Verification items for the finished model (mm, model axes). A direction names the side the tool comes from. Coordinates: 2 decimals unless noted, no trailing zeros. Loops run counter-clockwise (first coordinate to the right, second up) from the corner with the lowest first, then second, coordinate; pieces in that order, holes last. Notation, with made-up numbers: (73.5, 82) -> (118.5, 82) arc R12 cw to (118.5, 92) -> close; hole circle Ø11 at (38, -30). An arc over 180 degrees is marked (long way). Use CSV: the item, a comma, the result in double quotes. Start each with the question number.
```python
from build123d import *

# Parameters (mm, degrees)
AUFSATZ_LINEAR_AUSTRAGEN1_DEPTH            = 25
SCHNITT_LINEAR_AUSTRAGEN1_DEPTH            = 20
FASE1_SIZE                                 = 10
VERRUNDUNG1_R                              = 25
SKIZZE3_R                                  = 3.25
SCHNITT_LINEAR_AUSTRAGEN2_DEPTH            = 3.4
SKIZZE4_R                                  = 1.7
SCHNITT_LINEAR_AUSTRAGEN3_DEPTH            = 6.6
KREISMUSTER1_COUNT                         = 3
SKIZZE5_R                                  = 13
SCHNITT_LINEAR_AUSTRAGEN4_DEPTH            = 142.155942135
SKIZZE7_W                                  = 12
SKIZZE7_H                                  = 20
AUFSATZ_LINEAR_AUSTRAGEN2_DEPTH            = 10
SKIZZE9_R                                  = 1.7
SCHNITT_LINEAR_AUSTRAGEN7_DEPTH            = 78.781745931
SKIZZE8_R                                  = 3.25
SCHNITT_LINEAR_AUSTRAGEN6_DEPTH            = 3.4
SKIZZE10_R                                 = 13
SKIZZE10_R_2                               = 11
AUFSATZ_LINEAR_AUSTRAGEN3_DEPTH            = 2
SPIEGELN1_AT_THE_SECOND_PLANE_COPY_1_SKE_W = 12
SPIEGELN1_AT_THE_SECOND_PLANE_COPY_1_SKE_H = 20
SPIEGELN1_AT_THE_SECOND_PLANE_COPY_1_DEPTH = 10
SPIEGELN1_AT_THE_SECOND_PLANE_COPY_2_SKE_R = 1.7
SPIEGELN1_AT_THE_SECOND_PLANE_COPY_2_DEPTH = 78.781745931
SPIEGELN1_AT_THE_SECOND_PLANE_COPY_3_SKE_R = 3.25
SPIEGELN1_AT_THE_SECOND_PLANE_COPY_3_DEPTH = 3.4
SKIZZE11_R                                 = 1.9
SCHNITT_LINEAR_AUSTRAGEN8_DEPTH            = 10
KREISMUSTER2_COUNT                         = 4


with BuildPart() as part:
    # Skizze1 → Aufsatz-Linear austragen1 (new, symmetric)
    with BuildSketch(Plane(origin=(0, 0, 0), x_dir=(1, 0, 0), z_dir=(0, 1, 0))):
        Polygon((-60, 0), (60, 0), (60, -70), (48, -70), (48, -10), (-48, -10), (-48, -70), (-60, -70), align=None)
    extrude(amount=AUFSATZ_LINEAR_AUSTRAGEN1_DEPTH, both=True)

    # Skizze2 → Schnitt-Linear austragen1 (cut)
    with BuildSketch(Plane(origin=(0, 0, 0), x_dir=(-1, 0, 0), z_dir=(0, 0, -1))):
        with BuildLine():
            Line((-1.532970972, 2.1), (1.532970972, 2.1))
            ThreePointArc((1.532970972, 2.1), (0, -2.6), (-1.532970972, 2.1))
        make_face()
    extrude(amount=-SCHNITT_LINEAR_AUSTRAGEN1_DEPTH, mode=Mode.SUBTRACT)

    # Fase1
    fase1_edges = [part.edges().sort_by_distance(p)[0] for p in [
        (-60, 0, 0),
        (60, 0, 0),
        (48, 0, 10),
        (-48, 0, 10),
    ]]
    chamfer(fase1_edges, length=FASE1_SIZE)

    # Verrundung1
    verrundung1_edges = [part.edges().sort_by_distance(p)[0] for p in [
        (-54, -25, 70),
        (-54, 25, 70),
        (54, 25, 70),
        (54, -25, 70),
    ]]
    fillet(verrundung1_edges, radius=VERRUNDUNG1_R - 0.0001)  # a hair under: the kernel refuses the full size

    # Skizze3 → Schnitt-Linear austragen2 (cut)
    with BuildSketch(Plane.XY.offset(10)):
        with Locations((0, 12)):
            Circle(SKIZZE3_R)
    schnitt_linear_austragen2 = extrude(amount=-SCHNITT_LINEAR_AUSTRAGEN2_DEPTH, mode=Mode.SUBTRACT)

    # Skizze4 → Schnitt-Linear austragen3 (cut)
    with BuildSketch(Plane.XY.offset(6.6)):
        with Locations((0, 12)):
            Circle(SKIZZE4_R)
    schnitt_linear_austragen3 = extrude(amount=-SCHNITT_LINEAR_AUSTRAGEN3_DEPTH, mode=Mode.SUBTRACT)

    # Kreismuster1: Schnitt-Linear austragen2, Schnitt-Linear austragen3 ×3 about axis
    kreismuster1_axis = Axis((0, 0, 0), (0, 0, 1))
    add([schnitt_linear_austragen2.rotate(kreismuster1_axis, i * 360 / KREISMUSTER1_COUNT) for i in range(1, KREISMUSTER1_COUNT)], mode=Mode.SUBTRACT)
    add([schnitt_linear_austragen3.rotate(kreismuster1_axis, i * 360 / KREISMUSTER1_COUNT) for i in range(1, KREISMUSTER1_COUNT)], mode=Mode.SUBTRACT)

    # Skizze5 → Schnitt-Linear austragen4 (cut, through all)
    with BuildSketch(Plane(origin=(60, 0, 0), x_dir=(0, 0, -1), z_dir=(1, 0, 0))):
        with Locations((-45, 0)):
            Circle(SKIZZE5_R)
    extrude(amount=-SCHNITT_LINEAR_AUSTRAGEN4_DEPTH, mode=Mode.SUBTRACT)

    # Skizze7 → Aufsatz-Linear austragen2 (add, symmetric)
    with BuildSketch(Plane(origin=(0, 25, 0), x_dir=(1, 0, 0), z_dir=(0, 1, 0))):
        with Locations((-54, -45)):
            Rectangle(SKIZZE7_W, SKIZZE7_H)
    aufsatz_linear_austragen2 = extrude(amount=AUFSATZ_LINEAR_AUSTRAGEN2_DEPTH, both=True)

    # Skizze9 → Schnitt-Linear austragen7 (cut, through all)
    with BuildSketch(Plane.XY.offset(35)):
        with Locations((-54, 30)):
            Circle(SKIZZE9_R)
    schnitt_linear_austragen7 = extrude(amount=SCHNITT_LINEAR_AUSTRAGEN7_DEPTH, mode=Mode.SUBTRACT)

    # Skizze8 → Schnitt-Linear austragen6 (cut)
    with BuildSketch(Plane.XY.offset(55)):
        with Locations((-54, 30)):
            Circle(SKIZZE8_R)
    schnitt_linear_austragen6 = extrude(amount=-SCHNITT_LINEAR_AUSTRAGEN6_DEPTH, mode=Mode.SUBTRACT)

    # Skizze10 → Aufsatz-Linear austragen3 (add)
    with BuildSketch(Plane.ZY.offset(48)):
        with Locations(Location((45, 0, 0), (0, 0, 180))):
            Circle(SKIZZE10_R)
        with Locations((45, 0)):
            Circle(SKIZZE10_R_2, mode=Mode.SUBTRACT)
    extrude(amount=AUFSATZ_LINEAR_AUSTRAGEN3_DEPTH)

    # Spiegeln1: Aufsatz-Linear austragen2, Schnitt-Linear austragen7, Schnitt-Linear austragen6 across plane
    add(aufsatz_linear_austragen2.mirror(Plane(origin=(0, 0, 0), x_dir=(0, 0, 1), z_dir=(1, 0, 0))))
    add(schnitt_linear_austragen7.mirror(Plane(origin=(0, 0, 0), x_dir=(0, 0, 1), z_dir=(1, 0, 0))), mode=Mode.SUBTRACT)
    add(schnitt_linear_austragen6.mirror(Plane(origin=(0, 0, 0), x_dir=(0, 0, 1), z_dir=(1, 0, 0))), mode=Mode.SUBTRACT)

    # Spiegeln1 at the second plane: Aufsatz-Linear austragen2, Schnitt-Linear austragen7, Schnitt-Linear austragen6 across plane
    add(aufsatz_linear_austragen2.mirror(Plane.ZX))
    add(schnitt_linear_austragen7.mirror(Plane.ZX), mode=Mode.SUBTRACT)
    add(schnitt_linear_austragen6.mirror(Plane.ZX), mode=Mode.SUBTRACT)

    # Spiegeln1 at the second plane copy 1 ske → Spiegeln1 at the second plane copy 1 (add, symmetric)
    with BuildSketch(Plane(origin=(0, -25, 0), x_dir=(-1, 0, 0), z_dir=(0, -1, 0))):
        with Locations((-54, -45)):
            Rectangle(SPIEGELN1_AT_THE_SECOND_PLANE_COPY_1_SKE_W, SPIEGELN1_AT_THE_SECOND_PLANE_COPY_1_SKE_H)
    extrude(amount=SPIEGELN1_AT_THE_SECOND_PLANE_COPY_1_DEPTH, both=True)

    # Spiegeln1 at the second plane copy 2 ske → Spiegeln1 at the second plane copy 2 (cut, through all)
    with BuildSketch(Plane(origin=(0, 0, 35), x_dir=(-1, 0, 0), z_dir=(0, 0, 1))):
        with Locations((-54, 30)):
            Circle(SPIEGELN1_AT_THE_SECOND_PLANE_COPY_2_SKE_R)
    extrude(amount=SPIEGELN1_AT_THE_SECOND_PLANE_COPY_2_DEPTH, mode=Mode.SUBTRACT)

    # Spiegeln1 at the second plane copy 3 ske → Spiegeln1 at the second plane copy 3 (cut)
    with BuildSketch(Plane(origin=(0, 0, 55), x_dir=(-1, 0, 0), z_dir=(0, 0, 1))):
        with Locations((-54, 30)):
            Circle(SPIEGELN1_AT_THE_SECOND_PLANE_COPY_3_SKE_R)
    extrude(amount=-SPIEGELN1_AT_THE_SECOND_PLANE_COPY_3_DEPTH, mode=Mode.SUBTRACT)

    # Skizze11 → Schnitt-Linear austragen8 (cut)
    with BuildSketch(Plane(origin=(-60, 0, 0), x_dir=(0, 0, -1), z_dir=(1, 0, 0))):
        with Locations((-62.5, 0)):
            Circle(SKIZZE11_R)
    schnitt_linear_austragen8 = extrude(amount=SCHNITT_LINEAR_AUSTRAGEN8_DEPTH, mode=Mode.SUBTRACT)

    # Kreismuster2: Schnitt-Linear austragen8 ×4 about axis
    kreismuster2_axis = Axis((0, 0, 45), (1, 0, 0))
    for i in range(1, KREISMUSTER2_COUNT):
        add(schnitt_linear_austragen8.rotate(kreismuster2_axis, i * 360 / KREISMUSTER2_COUNT), mode=Mode.SUBTRACT)


solid = part.part
```
1. Cross-section at C-C, the plane y = 30. Record the boundary of the cut face in (x, z), plus the area to 3 significant figures.
2. Set-up check for faces 4 (the flat face through (-60, 8, 34)), 5 (the flat face through (1, 6, 10)), 6 (the cylindrical face through (-12.09, -5.93, 3.35)), 7 (the flat face through (-52.6, -28.6, 51.6)), 8 (the flat face through (-54, 32, 35)): record each of +Z, -Z, +X, -X, +Y, -Y from which the full face is reachable in a straight line by a thin tool's end or side.
3. Cross-section at A-A, the plane x = -54. State how many separate pieces and enclosed holes the cut face has, plus the area to 3 significant figures.
4. Scan lines: line 1 (X direction, y = -30, z = 45); line 2 (X direction, y = 4, z = 61); line 3 (X direction, y = -30, z = 53.1). Record each from-to range of solid material in increasing order.
5. Release check for a two-part mould opening along Y. For faces 1 (the cylindrical face through (-54.084, 13.862, 65.805)), 2 (the flat face through (-50, -3, 56)), 3 (the flat face through (-55, 0, 5)) record: released by +Y, released by -Y, zero draft, split by the parting line, or undercut.
6. Depth check by flat-ended pin: pin 1 (8 mm diameter, centred on x = 52.5, y = 29.5, fed in from -Z); pin 2 (4.5 mm diameter, centred on x = 0, y = 12, fed in from +Z); pin 3 (4 mm diameter, centred on x = 10.39, y = -6, fed in from -Z); pin 4 (15 mm diameter, centred on y = -2.5, z = 48.5, fed in from +X). Enter the tip coordinate at first touch or a pass-through.
7. Cross-section at D-D, the plane z = 16. Record the boundary of the cut face in (x, y).
Solution:
1,outline,"(-60, 35) -> (-55.7, 35) -> (-55.7, 51.6) -> (-57.25, 51.6) -> (-57.25, 55) -> (-60, 55) -> close; (-52.3, 35) -> (-48, 35) -> (-48, 55) -> (-50.75, 55) -> (-50.75, 51.6) -> (-52.3, 51.6) -> close; (48, 35) -> (52.3, 35) -> (52.3, 51.6) -> (50.75, 51.6) -> (50.75, 55) -> (48, 55) -> close; (55.7, 35) -> (60, 35) -> (60, 55) -> (57.25, 55) -> (57.25, 51.6) -> (55.7, 51.6) -> close"
1,area,"323 mm2"
2,face 4,"+Z, -Z, -X, +Y, -Y"
2,face 5,"+Z, +Y, -Y"
2,face 6,"+Z, -Z"
2,face 7,"+Z"
2,face 8,"-Z, +X, -X, +Y"
3,separate pieces,"3"
3,enclosed holes,"5"
3,area,"2,710 mm2"
4,line 1,"x = -60 to -55.7, -52.3 to -48, 48 to 52.3, 55.7 to 60"
4,line 2,"x = -60 to -48, 48 to 60"
4,line 3,"x = -60 to -57.25, -50.75 to -48, 48 to 50.75, 57.25 to 60"
5,face 1,"released by +Y"
5,face 2,"undercut"
5,face 3,"zero draft"
6,pin 1,"stops at z = 35"
6,pin 2,"stops at z = 6.6"
6,pin 3,"stops at z = 0"
6,pin 4,"stops at x = -48"
7,outline,"(-60, -25) -> (-44, -25) -> (-44, 25) -> (-60, 25) -> close; (44, -25) -> (60, -25) -> (60, 25) -> (44, 25) -> close"
